```python
from build123d import *

# Parameters (mm, degrees)
SKETCH1_R           = 25
SKETCH1_R_2         = 20.325
BOSS_EXTRUDE1_DEPTH = 20
BOSS_EXTRUDE2_START = -8
SKETCH1_2_R         = 25
BOSS_EXTRUDE2_DEPTH = 8
SKETCH3_W           = 12.4
SKETCH3_H           = 4.8
SKETCH3_R           = 1.325
CUT_EXTRUDE1_DEPTH  = 2.7
SKETCH3_4_W         = 12.4
SKETCH3_4_H         = 22.5
CUT_EXTRUDE3_DEPTH  = 44.7
SKETCH3_5_R         = 1.325
CUT_EXTRUDE4_DEPTH  = 38.7


with BuildPart() as part:
    # Sketch1 → Boss-Extrude1 (new body)
    with BuildSketch(Plane(origin=(0, 0, 0), x_dir=(1, 0, 0), z_dir=(0, 1, 0))):
        with Locations(Location((0, 0, 0), (0, 0, 270))):
            Circle(SKETCH1_R)
        with Locations(Location((0, 0, 0), (0, 0, 270))):
            Circle(SKETCH1_R_2, mode=Mode.SUBTRACT)
    extrude(amount=BOSS_EXTRUDE1_DEPTH)

    # Sketch1_2 → Boss-Extrude2 (add)
    with BuildSketch(Plane(origin=(0, 0, 0), x_dir=(1, 0, 0), z_dir=(0, 1, 0)).offset(BOSS_EXTRUDE2_START)):
        with Locations(Location((0, 0, 0), (0, 0, 270))):
            Circle(SKETCH1_2_R)
    extrude(amount=BOSS_EXTRUDE2_DEPTH)

    # Sketch3 → Cut-Extrude1 (cut)
    # profile 1 of 3: a face of its own
    with BuildSketch(Plane.XZ.offset(8)):
        with Locations((0, 18.7)):
            Rectangle(SKETCH3_W, SKETCH3_H)
        with Locations(Location((0, 18.7, 0), (0, 0, 270))):
            Circle(SKETCH3_R, mode=Mode.SUBTRACT)
    # profile 2 of 3: a face of its own
    with BuildSketch(Plane.XZ.offset(8)):
        with BuildLine():
            Line((6.2, -6.2), (0, -6.2))
            Line((0, -6.2), (0, -7.275))
            ThreePointArc((0, -7.275), (0.936916485, -7.663083515), (1.325, -8.6))
            ThreePointArc((1.325, -8.6), (0.936916485, -9.536916485), (0, -9.925))
            Line((0, -9.925), (0, -11))
            Line((0, -11), (6.2, -11))
            Line((6.2, -11), (6.2, -6.2))
        make_face()
    # profile 3 of 3: a face of its own
    with BuildSketch(Plane.XZ.offset(8)):
        with BuildLine():
            Line((0, -7.275), (0, -6.2))
            Line((0, -6.2), (-6.2, -6.2))
            Line((-6.2, -6.2), (-6.2, -11))
            Line((-6.2, -11), (0, -11))
            Line((0, -11), (0, -9.925))
            ThreePointArc((0, -9.925), (-1.325, -8.6), (0, -7.275))
        make_face()
    extrude(amount=-CUT_EXTRUDE1_DEPTH, mode=Mode.SUBTRACT)

    # Sketch3_4 → Cut-Extrude3 (cut)
    with BuildSketch(Plane.XZ.offset(8)):
        with Locations((0, 5.05)):
            Rectangle(SKETCH3_4_W, SKETCH3_4_H)
    extrude(amount=-CUT_EXTRUDE3_DEPTH, mode=Mode.SUBTRACT)

    # Sketch3_5 → Cut-Extrude4 (cut)
    with BuildSketch(Plane.XZ.offset(8)):
        with Locations(Location((0, 18.7, 0), (0, 0, 270))):
            Circle(SKETCH3_5_R)
        with BuildLine():
            ThreePointArc((1.325, -8.6), (0.936916485, -7.663083515), (0, -7.275))
            Line((0, -7.275), (0, -9.925))
            ThreePointArc((0, -9.925), (0.936916485, -9.536916485), (1.325, -8.6))
        make_face()
        with BuildLine():
            Line((0, -9.925), (0, -7.275))
            ThreePointArc((0, -7.275), (-1.325, -8.6), (0, -9.925))
        make_face()
    extrude(amount=-CUT_EXTRUDE4_DEPTH, mode=Mode.SUBTRACT)


solid = part.part
```
Check sheet for the modelled part. Datum: model origin and axes. Units: mm. A direction names the side the tool comes from. Round coordinates to 2 decimals unless told otherwise and drop trailing zeros. Loops run counter-clockwise (first coordinate to the right, second up) from the corner with the lowest first, then second, coordinate; pieces in that order, holes last. Notation, with made-up numbers: (0.25, 35) -> (56.25, 35) arc R14 ccw to (56.25, 50) -> close; hole circle Ø8 at (-12.5, 81.5). An arc over 180 degrees is marked (long way). Write item = value, one per line. Start each with the question number.
1) Release check for a two-part mould opening along Z. For faces 4 (the flat face through (-11, -8, 0)), 5 (the flat face through (6.2, -4, 5)), 6 (the cylindrical face through (7.509, 5.804, 23.846)) record: released by +Z, released by -Z, zero draft, split by the parting line, or undercut.
2) Set-up check for faces 1 (the cylindrical face through (6.105, 9.86, 19.386)), 2 (the flat face through (-1.5, -5.3, -8.6)), 3 (the flat face through (0, -3, -6.2)): record each of +Z, -Z, +X, -X, +Y, -Y from which the full face is reachable in a straight line by a thin tool's end or side.
3) Sectioned sample at C-C, the plane y = 5.25. Record the cut outline in (x, z) (3 decimals).
4) Thickness scan on probe 1 along X at (y, z) = (10, 0) (3 decimals); probe 2 along Y at (x, z) = (-11, 6); probe 3 along Y at (x, z) = (6, 20). Record the ranges inside material, lowest first.
5) Sectioned sample at D-D, the plane z = 18.7. Record the cut outline in (x, y) (3 decimals).
6) Sectioned sample at A-A, the plane z = 0. Record the cut outline in (x, y) (3 decimals), plus the area to 3 significant figures.
7) Sectioned sample at B-B, the plane x = 5.5. Record the cut outline in (y, z), plus the area to 3 significant figures.
8) Gauge pin test, flat ends, axial feed: pin 1 Ø2.5 at (y, z) = (-4, 12) entering from -X; pin 2 Ø2.5 at (x, y) = (-0.5, -3) entering from -Z; pin 3 Ø3 at (x, y) = (4, 14.5) entering from -Z; pin 4 Ø2.5 at (x, z) = (2, -8.5) entering from -Y. Record the tip position at first contact, or that the pin passes through.
Results are:
q1.face_4 = zero draft
q1.face_5 = undercut
q1.face_6 = split by the parting line
q2.face_1 = +Y
q2.face_2 = -Y
q2.face_3 = +Y, -Y
q3.outline = circle Ø50 at (0, 0); hole circle Ø40.65 at (0, 0)
q4.probe_1 = -25 to -20.325, 20.325 to 25
q4.probe_2 = -8 to 0
q4.probe_3 = -5.3 to 20
q5.outline = (-16.592, -8) -> (-6.2, -8) -> (-6.2, -5.3) -> (-1.325, -5.3) -> (-1.325, 0) -> (-7.963, 0) -> (-7.963, 20) -> (-16.592, 20) -> close; (1.325, -5.3) -> (6.2, -5.3) -> (6.2, -8) -> (16.592, -8) -> (16.592, 20) -> (7.963, 20) -> (7.963, 0) -> (1.325, 0) -> close
q6.outline = (-25, -8) -> (-6.2, -8) -> (-6.2, 0) -> (-20.325, 0) -> (-20.325, 20) -> (-25, 20) -> close; (6.2, -8) -> (25, -8) -> (25, 20) -> (20.325, 20) -> (20.325, 0) -> (6.2, 0) -> close
q6.area = 488 mm^2
q7.outline = (-8, -24.39) -> (20, -24.39) -> (20, -19.57) -> (0, -19.57) -> (0, -6.2) -> (-5.3, -6.2) -> (-5.3, -11) -> (-8, -11) -> close; (-8, 21.1) -> (-5.3, 21.1) -> (-5.3, 16.3) -> (0, 16.3) -> (0, 19.57) -> (20, 19.57) -> (20, 24.39) -> (-8, 24.39) -> close
q7.area = 377 mm^2
q8.pin_1 = -22.57
q8.pin_2 = -25
q8.pin_3 = -24.87
q8.pin_4 = -5.3
